Check sheet for the modelled part. Datum: model origin and axes. Units: mm. A direction names the side the tool comes from. Round coordinates to 2 decimals unless told otherwise and drop trailing zeros. Order: outer loops, then holes, each group sorted by start corner. A loop starts at its lowest first (then second) coordinate and runs counter-clockwise, first axis right, second up.
Autodesk Inventor part; units mm, degrees
ref_plane "YZ Plane" through (0, 0, 0) normal (1, 0, 0) x (0, 1, 0)
ref_plane "XZ Plane" through (0, 0, 0) normal (0, 1, 0) x (-1, 0, 0)
ref_plane "XY Plane" through (0, 0, 0) normal (0, 0, 1) x (1, 0, 0)
sketch "Sketch1" plane through (0, 0, 0) normal (0, 1, 0) x (-1, 0, 0)
  arc A0 (10.8783, 63.6799) -> (10.8783, -82.6701) centre (10.8783, -9.4951) ccw
  line L0 (10.8783, 63.6799) -> (40.8783, 63.6799)
  line L1 (40.8783, -82.6701) -> (10.8783, -82.6701)
  line L2 (40.8783, -79.4951) -> (10.8783, -79.4951)
  arc A1 (10.8783, 60.5049) -> (10.8783, -79.4951) centre (10.8783, -9.4951) ccw
  line L3 (10.8783, 60.5049) -> (40.8783, 60.5049)
  line L4 (40.8783, 63.6799) -> (40.8783, 60.5049)
  line L5 (40.8783, -79.4951) -> (40.8783, -82.6701)
  line L6 (25.8783, -82.6701) -> (25.8783, -9.4951)
  line L7 (25.8783, -9.4951) -> (10.8783, -9.4951)
  dimension "d1" = 30
  dimension "d2" = 3.175
  dimension "d15" = 70
extrude "Extrusion1" add sketch "Sketch1" along normal blind 40
sketch "Sketch2" plane through (-40.8783, 0, 63.6799) normal (0, 0, 1) x (1, 0, 0)
  line L0 (29.9701, 0) -> (0, 40)
  line L1 (0, 40) -> (30, 40)
  line L2 (0, 40) -> (30, 40)
  line L3 (30, 40) -> (0, 0)
  circle A0 centre (15, 20) radius 6
  point P0 (40.8783, 0)
  dimension "d5" = 12
extrude "Extrusion2" cut sketch "Sketch2" against normal blind 200 contours A0 L3 L0 | L0 L3 A0 | L3 A0 L0 | L0 A0 L3
fillet "Fillet1" radius 10 2 edges at (-40.8783, 40, 62.0924) (-40.8783, 0, 62.0924)
fillet "Fillet2" radius 10 2 edges at (-40.8783, 40, -81.0826) (-40.8783, 0, -81.0826)
sketch "Sketch3" plane through (-40.8783, 10, -79.4951) normal (-1, 0, 0) x (0, 0, 1)
  line L0 (-3.175, 0) -> (143.175, 20)
  line L1 (143.175, -10) -> (143.175, 30)
  line L2 (143.175, 0) -> (-3.175, 20)
  circle A0 centre (70, 10) radius 6
  point P0 (79.4951, -10)
  dimension "d10" = 12
extrude "Extrusion3" cut sketch "Sketch3" against normal blind 200 contours A0 L2 L0 | L0 L2 A0 | L2 A0 L0 | L0 A0 L2
properties part number "APOIO_TUBO"
1) Scan lines: line 1 (Z direction, x = -26.5, y = 3); line 2 (Z direction, x = 13.5, y = 18); line 3 (X direction, y = 27, z = -10). Record each from-to range of solid material in increasing order.
2) Draft check along X on faces 1 (the face through (-19, 20, 60.505)), 2 (the face through (-20.155, 21.802, 62.115)), 3 (the face through (-38.03, 36.99, 62.07)). Enter one of: pulls with the +X half, pulls with the -X half, needs draft (parallel to the pull), parting line crosses it, or undercut.
3) Sectioned sample at D-D on x = -5.5. Record the cut outline in (y, z).
4) Sectioned sample at C-C on y = 33.5. Record the cut outline in (x, z) (3 decimals).
5) Sectioned sample at B-B on x = 31. Record the cut outline in (y, z).
6) Gauge pin test, flat ends, axial feed: pin 1 (4 mm diameter, centred on y = 7.5, z = 8.5, fed in from +X); pin 2 (2 mm diameter, centred on x = 18.5, y = 32, fed in from +Z); pin 3 (4 mm diameter, centred on x = 29.5, y = 13, fed in from +Z). Record the tip position at first contact, or that the pin passes through.
7) Sectioned sample at A-A on y = 16. Record the cut outline in (x, z) (3 decimals).
8) Set-up check for faces 4 (the face through (-20.155, 21.802, -81.06)), 5 (the face through (-19, 20, -79.495)): record each of +Z, -Z, +X, -X, +Y, -Y from which the full face is reachable in a straight line by a thin tool's end or side.
Values found:
1. line 1: z = -82.67 to -79.5, 60.5 to 63.68
1. line 2: z = -78.49 to -75.11, 56.12 to 59.5
1. line 3: x = 59.12 to 62.29
2. face 1: needs draft
2. face 2: undercut
2. face 3: pulls with the -X half
3. outline: (0, -82.47) - (40, -82.47) - (40, -79.29) - (0, -79.29) - close; (0, 60.3) - (40, 60.3) - (40, 63.48) - (0, 63.48) - close
4. outline: (-40.246, -82.67) - (-10.878, -82.67) arc R73.175 ccw to (-10.878, 63.68) - (-40.246, 63.68) - (-40.246, 60.505) - (-10.878, 60.505) arc R70 cw to (-10.878, -79.495) - (-40.246, -79.495) - close
5. outline: (0, -69.5) - (40, -69.5) - (40, -65.59) - (0, -65.59) - close; (0, 46.6) - (40, 46.6) - (40, 50.51) - (0, 50.51) - close
6. pin 1: stops at x = 60.53
6. pin 2: stops at z = 57.95
6. pin 3: stops at z = 52.81
7. outline: (-40.878, -82.67) - (-30.35, -82.67) - (-30.35, -79.495) - (-40.878, -79.495) - close; (-40.878, 60.505) - (-30.35, 60.505) - (-30.35, 63.68) - (-40.878, 63.68) - close; (-21.406, -82.67) - (-10.878, -82.67) arc R73.175 ccw to (62.16, -13.967) - (58.979, -13.967) arc R70 cw to (-10.878, -79.495) - (-21.406, -79.495) - close; (-21.406, 60.505) - (-10.878, 60.505) arc R70 cw to (58.979, -5.023) - (62.16, -5.023) arc R73.175 ccw to (-10.878, 63.68) - (-21.406, 63.68) - close
8. face 4: +Z, -Z
8. face 5: -X, +Y, -Y
